For this review, take the finished solid that the model builds, in its own axes (mm). A direction names the side the tool comes from. Coordinates: 2 decimals unless noted, no trailing zeros.
```python
from build123d import *

# Parameters (mm, degrees)
F0_R     = 62.5
F1_DEPTH = 30
F2_SIZE  = 25
F3_R     = 6.65
F4_DEPTH = 25
F5_R     = 5
F6_R     = 5
F7_R     = 45
F7_R_2   = 22.5
F8_DEPTH = 10
F9_SIZE  = 5


with BuildPart() as f1:
    # F0 (on Top) → F1 (new body)
    with BuildSketch(Plane.XY):
        Circle(F0_R)
    extrude(amount=F1_DEPTH)

    # F2
    f2_edges = [f1.edges().sort_by_distance(p)[0] for p in [
        (-62.5, 0, 30),
    ]]
    chamfer(f2_edges, length=F2_SIZE)

    # F3 (on face) → F4 (cut)
    with BuildSketch(Plane.XY.offset(30)):
        Circle(F3_R)
    extrude(amount=-F4_DEPTH, mode=Mode.SUBTRACT)

    # F5
    f5_edges = [f1.edges().sort_by_distance(p)[0] for p in [
        (-37.5, 0, 30),
    ]]
    fillet(f5_edges, radius=F5_R)

    # F6
    f6_edges = [f1.edges().sort_by_distance(p)[0] for p in [
        (-62.5, 0, 5),
    ]]
    fillet(f6_edges, radius=F6_R)

    # F7 (on face) → F8 (cut)
    with BuildSketch(Plane(origin=(0, 0, 0), x_dir=(1, 0, 0), z_dir=(0, 0, -1))):
        Circle(F7_R)
        Circle(F7_R_2, mode=Mode.SUBTRACT)
    extrude(amount=-F8_DEPTH, mode=Mode.SUBTRACT)

    # F9
    f9_edges = [f1.edges().sort_by_distance(p)[0] for p in [
        (-45, 0, 0),
        (-22.5, 0, 0),
    ]]
    chamfer(f9_edges, length=F9_SIZE)


solid = f1.part
```
Q1. For probe 1 along Y at (x, z) = (0, 7.45); probe 2 along Y at (x, z) = (0, 6.7); probe 3 along Z at (x, y) = (-25, 10), list the stretches that pass through material, from the lowest coordinate up.
Ans:
probe 1: y = -60.05 to -45, -22.5 to -6.65, 6.65 to 22.5, 45 to 60.05
probe 2: y = -60.8 to -45, -22.5 to -6.65, 6.65 to 22.5, 45 to 60.8
probe 3: z = 10 to 30
Q2. Tool access review of faces 1 (the flat face through (9, -21, 10)), 2 (the flat face through (0, 0, 5)), 3 (the flat face through (0, 0, 0)): name each direction out of +Z, -Z, +X, -X, +Y, -Y from which nothing blocks a thin tool from reaching the whole face with its end or side.
Ans:
face 1: -Z
face 2: +Z
face 3: -Z, +X, -X, +Y, -Y
Q3. Draft analysis for pull direction X (two halves, no side actions). For faces 4 (the conical face through (41.79, 17.33, 4.76)), 5 (the cylindrical face through (10.382, 19.961, 7.465)), 6 (the cylindrical face through (57.734, -23.938, 1.444)), 7 (the flat face through (0, -7, 30)), state which applies: +X half, -X half, draft (parallel to the pull), parting line (faces both ways), or undercut.
Ans:
face 4: undercut
face 5: undercut
face 6: parting line
face 7: draft
Q4. Clearance check with flat-ended pins moving along their axes: pin 1 Ø2 at (y, z) = (-42.5, 8) entering from -X; pin 2 Ø1 at (y, z) = (1, 20.5) entering from -X; pin 3 Ø3 at (x, y) = (22.5, -30) entering from -Z. State where each tip first meets the part, or that it passes through.
Ans:
pin 1: stops at x = -43.37
pin 2: stops at x = -47.49
pin 3: stops at z = 10
